```python
from build123d import *

# Parameters (mm, degrees)
SZKIC1_R                    = 11.5
DODANIE_WYCI_GNI_CIE1_DEPTH = 3
SZKIC2_R                    = 4
DODANIE_WYCI_GNI_CIE2_DEPTH = 9
SZKIC3_R                    = 1.5
WYTNIJ_WYCI_GNI_CIE1_DEPTH  = 2
DODANIE_WYCI_GNI_CIE3_DEPTH = 3
DODANIE_WYCI_GNI_CIE4_DEPTH = 30
ZAOKR_GLENIE1_R             = 10
ZAOKR_GLENIE2_R             = 30
ZAOKR_GLENIE6_R             = 1
ZAOKR_GLENIE8_R             = 0.5
ZAOKR_GLENIE9_R             = 0.5


with BuildPart() as part:
    # Szkic1 → Dodanie-wyciągnięcie1 (new body)
    with BuildSketch(Plane.XY):
        with Locations((68.25, -14)):
            Circle(SZKIC1_R)
    extrude(amount=DODANIE_WYCI_GNI_CIE1_DEPTH)

    # Szkic2 → Dodanie-wyciągnięcie2 (add)
    with BuildSketch(Plane(origin=(0, 0, 0), x_dir=(-1, 0, 0), z_dir=(0, 0, -1))):
        with Locations((-68.25, -14)):
            Circle(SZKIC2_R)
    extrude(amount=DODANIE_WYCI_GNI_CIE2_DEPTH)

    # Szkic3 → Wytnij-wyciągnięcie1 (cut)
    with BuildSketch(Plane.XY.offset(3)):
        with Locations((74.000947528, -19.561169169)):
            Circle(SZKIC3_R)
        with Locations((73.811169169, -8.249052472)):
            Circle(SZKIC3_R)
        with Locations((62.499052472, -8.438830831)):
            Circle(SZKIC3_R)
        with Locations((62.688830831, -19.750947528)):
            Circle(SZKIC3_R)
    extrude(amount=-WYTNIJ_WYCI_GNI_CIE1_DEPTH, mode=Mode.SUBTRACT)

    # Szkic4 → Dodanie-wyciągnięcie3 (add)
    with BuildSketch(Plane.XY.offset(3)):
        Polygon((68.25, -2.5), (128.25, -2.5), (141.25, -14), (141.25, -25.5), (136.25, -25.5), (136.25, -17.31662479), (128.25, -9.5), (98.25, -9.5), (77.80017301, -20.406574394), (76.895320055, -6.416567983), align=None)
    extrude(amount=-DODANIE_WYCI_GNI_CIE3_DEPTH)

    # Szkic6 → Dodanie-wyciągnięcie4 (add)
    with BuildSketch(Plane(origin=(0, 0, 0), x_dir=(-1, 0, 0), z_dir=(0, 0, -1))):
        Polygon((-82.25, -2.5), (-128.25, -2.5), (-141.25, -14), (-141.25, -25.5), (-136.25, -25.5), (-136.25, -24.5), (-139.75, -24.5), (-139.75, -14.901008455), (-127.489427722, -4.5), (-82.25, -4.5), align=None)
    extrude(amount=DODANIE_WYCI_GNI_CIE4_DEPTH)

    # Zaokrąglenie1
    zaokr_glenie1_edges = [part.edges().sort_by_distance(p)[0] for p in [
        (128.25, -2.5, -13.5),
        (141.25, -14, -13.5),
        (136.25, -17.31662479, 1.5),
        (128.25, -9.5, 1.5),
        (139.75, -14.901008455, -15),
        (127.489427722, -4.5, -15),
    ]]
    fillet(zaokr_glenie1_edges, radius=ZAOKR_GLENIE1_R)

    # Zaokrąglenie2
    zaokr_glenie2_edges = [part.edges().sort_by_distance(p)[0] for p in [
        (98.25, -9.5, 1.5),
    ]]
    fillet(zaokr_glenie2_edges, radius=ZAOKR_GLENIE2_R)

    # Zaokrąglenie6
    zaokr_glenie6_edges = [part.edges().sort_by_distance(p)[0] for p in [
        (141.25, -25.5, -13.5),
        (139.75, -24.5, -15),
        (82.25, -2.5, -15),
        (82.25, -4.5, -15),
    ]]
    fillet(zaokr_glenie6_edges, radius=ZAOKR_GLENIE6_R - 0.0001)  # a hair under: the kernel refuses the full size

    # Zaokrąglenie8
    zaokr_glenie8_edges = [part.edges().sort_by_distance(p)[0] for p in [
        (136.25, -25.5, -13.5),
        (136.25, -24.5, -15),
    ]]
    fillet(zaokr_glenie8_edges, radius=ZAOKR_GLENIE8_R - 0.0001)  # a hair under: the kernel refuses the full size

    # Zaokrąglenie9
    zaokr_glenie9_edges = [part.edges().sort_by_distance(p)[0] for p in [
        (141.25, -21.502571138, -30),
        (140.36749385, -14.397572751, -30),
        (128.004313516, -3.148538717, -30),
        (138.824438517, -15.329570819, -30),
        (127.264686983, -5.112328638, -30),
        (103.855795671, -2.5, -30),
        (138.5, -25.5, -30),
        (139.75, -21.515702231, -30),
        (140.957136071, -25.207136071, -30),
        (82.542863929, -4.207136071, -30),
        (82.542863929, -2.792863929, -30),
        (139.457136071, -24.207136071, -30),
        (137.75, -24.5, -30),
        (136.39641732, -24.64641732, -30),
        (136.39641732, -25.35358268, -30),
        (133.253669041, -9.38997751, -30),
        (103.534532162, -4.5, -30),
        (134.481584493, -8.012555513, -30),
    ]]
    fillet(zaokr_glenie9_edges, radius=ZAOKR_GLENIE9_R - 0.0001)  # a hair under: the kernel refuses the full size


solid = part.part
```
For this review, take the finished solid that the model builds, in its own axes (mm). A direction names the side the tool comes from. Give positions to 0.01 mm unless a question says otherwise; leave off trailing zeros. Order: outer loops, then holes, each group sorted by start corner. A loop starts at its lowest first (then second) coordinate and runs counter-clockwise, first axis right, second up.
1) Insertion check: pin 1 (1 mm diameter, centred on y = -10, z = -3.5, fed in from -X); pin 2 (4.5 mm diameter, centred on y = -21.5, z = -16.5, fed in from -X); pin 3 (2.5 mm diameter, centred on x = 74, y = -19.56, fed in from -Z). Each pin has a flat end and moves straight along its axis. Give the tip position at first contact, or say it passes through.
2) Wall thickness on line 1 (Z direction, x = 68.5, y = -9); line 2 (X direction, y = -23.5, z = 0.5); line 3 (Y direction, x = 106, z = -23): over which ranges is each line inside the solid? List them lowest first.
3) Take a section at D-D (x = 102). Give the boundary of the cut face in (y, z).
4) The part is to be moulded in two halves that separate along Y. For faces 5 (the face through (134.434, -7.971, -13.023)), 6 (the face through (61, -8.4, 2)), 7 (the face through (74.618, -6.984, 2.014)), 8 (the face through (132.22, -13.38, 1.52)), say which applies: released by +Y, released by -Y, zero draft, split by the parting line, or undercut.
5) Take a section at B-B (x = 116). Give the boundary of the cut face in (y, z), then the cut area to 3 significant figures.
6) For faces 1 (the face through (102, -2.5, -13)), 2 (the face through (74, -20, 1)), 3 (the face through (135.49, -17.7, 1.48)), 4 (the face through (127.218, -5.095, -14.957)), list the 3-axis set-ups (+Z, -Z, +X, -X, +Y, -Y) from which the entire face can be reached by the end or side of a thin tool; tool diameter is ignored.
Derived:
1. pin 1: stops at x = 66.31
1. pin 2: stops at x = 139.72
1. pin 3: stops at z = 0
2. line 1: z = 0 to 3
2. line 2: x = 61.77 to 74.73, 136.25 to 141.25
2. line 3: y = -4.5 to -2.5
3. outline: (-9.74, 0) - (-4.5, 0) - (-4.5, -29.5) arc R0.5 ccw to (-4, -30) - (-3, -30) arc R0.5 ccw to (-2.5, -29.5) - (-2.5, 3) - (-9.74, 3) - close
4. face 5: released by +Y
4. face 6: undercut
4. face 7: undercut
4. face 8: released by -Y
5. outline: (-9.5, 0) - (-4.5, 0) - (-4.5, -29.5) arc R0.5 ccw to (-4, -30) - (-3, -30) arc R0.5 ccw to (-2.5, -29.5) - (-2.5, 3) - (-9.5, 3) - close
5. area: 80.9 mm2
6. face 1: +Z, -Z, +X, -X, +Y
6. face 2: +Z
6. face 3: +Z, -Z, -Y
6. face 4: -Z, -X, -Y
